from build123d import *

# Parameters (mm, degrees)
SKETCH1_W           = 13.97
SKETCH1_H           = 12.7
BOSS_EXTRUDE1_DEPTH = 2.54
FILLET1_R           = 0.635
SHELL1_START        = 0.635
SHELL1_OUTLINE_W    = 1.905
SHELL1_OUTLINE_H    = 11.43
SHELL1_DEPTH        = 12.7
SKETCH2_R           = 2.54
BOSS_EXTRUDE2_DEPTH = 1.905
SKETCH3_W           = 0.569871795
SKETCH3_H           = 3.256410256
BOSS_EXTRUDE3_DEPTH = 0.00254


# Read off the part's stored shape, not the designer's step: Shell1
with BuildPart() as part:
    # Sketch1 → Boss-Extrude1 (new body)
    with BuildSketch(Plane(origin=(0, 0, 0), x_dir=(1, 0, 0), z_dir=(0, 1, 0))):
        with Locations((6.985, 6.35)):
            Rectangle(SKETCH1_W, SKETCH1_H)
    extrude(amount=BOSS_EXTRUDE1_DEPTH)

    # Fillet1
    fillet1_edges = [part.edges().sort_by_distance(p)[0] for p in [
        (0, 1.27, -12.7),
        (13.97, 1.27, -12.7),
        (13.97, 1.27, 0),
        (0, 1.27, 0),
    ]]
    fillet(fillet1_edges, radius=FILLET1_R)

    # Shell1 outline → Shell1 (cut)
    with BuildSketch(Plane.YZ.offset(SHELL1_START)):
        with Locations((0.9525, -6.35)):
            Rectangle(SHELL1_OUTLINE_W, SHELL1_OUTLINE_H)
    extrude(amount=SHELL1_DEPTH, mode=Mode.SUBTRACT)

    # Sketch2 → Boss-Extrude2 (add)
    with BuildSketch(Plane(origin=(0, 1.905, 0), x_dir=(-1, 0, 0), z_dir=(0, -1, 0))):
        with Locations(Location((-6.985, 6.35, 0), (0, 0, 270))):
            Circle(SKETCH2_R)
    extrude(amount=BOSS_EXTRUDE2_DEPTH)

    # Sketch3 → Boss-Extrude3 (add)
    # profile 1 of 3: a face of its own
    with BuildSketch(Plane(origin=(0, 2.54, 0), x_dir=(1, 0, 0), z_dir=(0, 1, 0))):
        Polygon((5.026905248, 8.255), (5.555435897, 8.255), (6.837647436, 5.08), (6.228978566, 5.08), (5.982203726, 5.731282051), (4.598865385, 5.731282051), (4.352090545, 5.08), (3.744057692, 5.08), align=None)
        Polygon((5.290852564, 7.403372396), (4.815111378, 6.301153846), (5.76659375, 6.301153846), align=None, mode=Mode.SUBTRACT)
    # profile 2 of 3: a face of its own
    with BuildSketch(Plane(origin=(0, 2.54, 0), x_dir=(1, 0, 0), z_dir=(0, 1, 0))):
        with Locations((7.468576924, 6.708205128)):
            Rectangle(SKETCH3_W, SKETCH3_H)
    # profile 3 of 3: a face of its own
    with BuildSketch(Plane(origin=(0, 2.54, 0), x_dir=(1, 0, 0), z_dir=(0, 1, 0))):
        Polygon((8.323384615, 8.336410256), (8.89325641, 8.336410256), (8.89325641, 7.400192308), (9.259602564, 7.400192308), (9.259602564, 6.911730769), (8.89325641, 6.911730769), (8.89325641, 5.08), (8.323384615, 5.08), (8.323384615, 6.911730769), (8.038448718, 6.911730769), (8.038448718, 7.400192308), (8.323384615, 7.400192308), align=None)
    extrude(amount=BOSS_EXTRUDE3_DEPTH)


solid = part.part
Source: CAD feature listing. Evaluate the final solid. Frame: model axes, mm. A direction names the side the tool comes from. Give positions to 0.01 mm unless a question says otherwise; leave off trailing zeros. Write each loop counter-clockwise with the first axis right and the second up, starting at its lowest first coordinate (ties: lowest second). Pieces come first, ordered by that corner, then holes. Notation, with made-up numbers: (6.25, 89.25) - (63.25, 89.25) arc R20 cw to (63.25, 94.25) - close; hole circle Ø11 at (43.5, 41). An arc over 180 degrees is marked (long way). Write item = value, one per line. Start each with the question number.
Q1. Cut plane A-A, the plane z = -10.75. Return loops of the section in (x, y) (3 decimals).
Q2. Material intervals for probe 1 along X at (y, z) = (1.35, -11) (3 decimals); probe 2 along Z at (x, y) = (5.75, 1.3) (3 decimals); probe 3 along Z at (x, y) = (13, 1.65) (3 decimals), sorted ascending.
Q3. Cut plane B-B, the plane x = 10.5. Return loops of the section in (y, z) (3 decimals), then the cut area to 3 significant figures.
Q4. Draft query along Z for faces 3 (the flat face through (7, 1, 0)), 4 (the flat face through (8.7, 2.543, -6.7)), 5 (the flat face through (0.635, 1, -6)), 6 (the flat face through (7, 1, -12.7)). Return one class per face: +Z half, -Z half, draft (parallel to the pull), parting line (faces both ways), or undercut.
Q5. Reachability of faces 1 (the flat face through (6.4, 0, -0.3)), 2 (the flat face through (13.335, 1, -6)) from +Z, -Z, +X, -X, +Y, -Y: full face, straight path, thin tool, end or side. Return the list, or none.
Q6. Cut plane C-C, the plane z = -8.5. Return loops of the section in (x, y) (3 decimals).
Computed values:
q1.outline = (0, 0) - (0.635, 0) - (0.635, 1.905) - (13.335, 1.905) - (13.335, 0) - (13.97, 0) - (13.97, 2.54) - (0, 2.54) - close
q2.probe_1 = 0 to 0.635, 13.335 to 13.97
q2.probe_2 = -12.7 to -12.065, -8.57 to -4.13, -0.635 to 0
q2.probe_3 = -12.7 to -12.065, -0.635 to 0
q3.outline = (0, -12.7) - (2.54, -12.7) - (2.54, 0) - (0, 0) - (0, -0.635) - (1.905, -0.635) - (1.905, -12.065) - (0, -12.065) - close
q3.area = 10.5 mm²
q4.face_3 = +Z half
q4.face_4 = draft
q4.face_5 = undercut
q4.face_6 = -Z half
q5.face_1 = +Z, -Z, +X, -X, -Y
q5.face_2 = -Y
q6.outline = (0, 0) - (0.635, 0) - (0.635, 1.905) - (5.633, 1.905) - (5.633, 0) - (8.337, 0) - (8.337, 1.905) - (13.335, 1.905) - (13.335, 0) - (13.97, 0) - (13.97, 2.54) - (0, 2.54) - close
